Could you check a few things on this drawing? It's one solid part, dimensions in mm from its lowest x, y, z. A direction names the side the tool comes from. Round coordinates to 2 decimals unless told otherwise and drop trailing zeros. Order: outer loops, then holes, each group sorted by start corner. A loop starts at its lowest first (then second) coordinate and runs counter-clockwise, first axis right, second up.
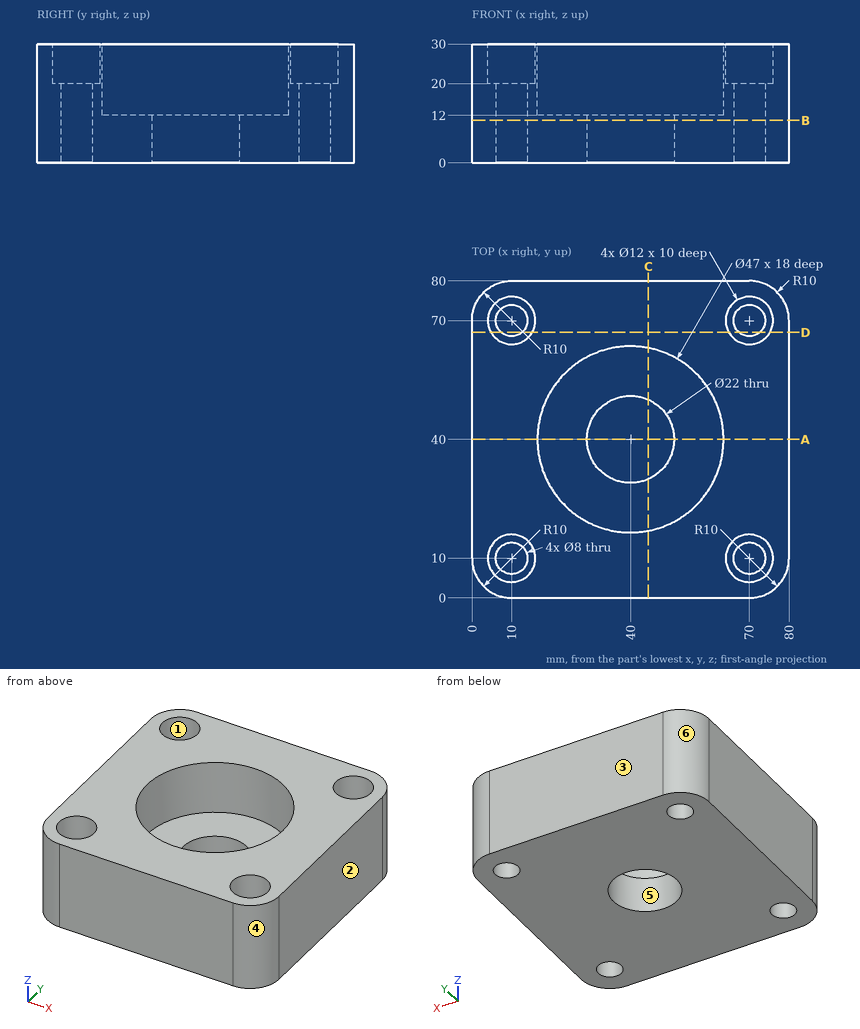
1) If we section it at D-D (y = 67): Write out the boundary of the cut face in (x, z), plus the area to 3 significant figures.
2) If we section it at A-A (y = 40): Write out the boundary of the cut face in (x, z).
3) For the marked faces 1 and 2, which set-ups out of +Z, -Z, +X, -X, +Y, -Y let a thin tool reach every point of the face, with its end or its side?
4) If we section it at C-C (x = 44.5): Write out the boundary of the cut face in (y, z).
5) I need wall thicknesses on line 1 (Y direction, x = 70, z = 14); line 2 (Y direction, x = 10, z = 26.25); line 3 (X direction, y = 41, z = 25.75). Which ranges of each line are inside material? Lowest first, please.
6) If we section it at B-B (z = 10.75): Write out the boundary of the cut face in (x, y), plus the area to 3 significant figures.
7) We'd pull the mould along X, two halves only. Please class the marked faces 3, 4, 5 and 6: +X half, -X half, draft (parallel to the pull), parting line (faces both ways), or undercut.
8) I'm going to push flat-ended pins straight in: pin 1 (3.5 mm diameter, centred on x = 11.5, y = 7, fed in from +Z); pin 2 (6.5 mm diameter, centred on x = 10, y = 10, fed in from +Z); pin 3 (3 mm diameter, centred on x = 71, z = 3, fed in from -Y). Where does each tip first touch, or does it pass through?
Solutions:
1. outline: (0, 0) - (7.35, 0) - (7.35, 20) - (4.8, 20) - (4.8, 30) - (0, 30) - close; (12.65, 0) - (67.35, 0) - (67.35, 20) - (64.8, 20) - (64.8, 30) - (15.2, 30) - (15.2, 20) - (12.65, 20) - close; (72.65, 0) - (80, 0) - (80, 30) - (75.2, 30) - (75.2, 20) - (72.65, 20) - close
1. area: 1,980 mm2
2. outline: (0, 0) - (29, 0) - (29, 12) - (16.5, 12) - (16.5, 30) - (0, 30) - close; (51, 0) - (80, 0) - (80, 30) - (63.5, 30) - (63.5, 12) - (51, 12) - close
3. face 1: +Z
3. face 2: +Z, -Z, +X, +Y, -Y
4. outline: (0, 0) - (29.96, 0) - (29.96, 12) - (16.93, 12) - (16.93, 30) - (0, 30) - close; (50.04, 0) - (80, 0) - (80, 30) - (63.07, 30) - (63.07, 12) - (50.04, 12) - close
5. line 1: y = 0 to 6, 14 to 66, 74 to 80
5. line 2: y = 0 to 4, 16 to 64, 76 to 80
5. line 3: x = 0 to 16.52, 63.48 to 80
6. outline: (0, 10) arc R10 ccw to (10, 0) - (70, 0) arc R10 ccw to (80, 10) - (80, 70) arc R10 ccw to (70, 80) - (10, 80) arc R10 ccw to (0, 70) - close; hole circle Ø8 at (10, 10); hole circle Ø8 at (10, 70); hole circle Ø22 at (40, 40); hole circle Ø8 at (70, 10); hole circle Ø8 at (70, 70)
6. area: 5,730 mm2
7. face 3: draft
7. face 4: +X half
7. face 5: undercut
7. face 6: -X half
8. pin 1: stops at z = 20
8. pin 2: passes through
8. pin 3: stops at y = 0
